Check sheet for the modelled part. Datum: model origin and axes. Units: mm. Face numbers are marked on the shaded views. Round coordinates to 2 decimals unless told otherwise and drop trailing zeros. Order: outer loops, then holes, each group sorted by start corner. A loop starts at its lowest first (then second) coordinate and runs counter-clockwise, first axis right, second up.
from build123d import *

# Parameters (mm, degrees)
SKETCH1_R           = 62.5
SKETCH1_R_2         = 33.5
BOSS_EXTRUDE1_DEPTH = 30
SKETCH2_W           = 16
SKETCH2_H           = 6.75
CUT_EXTRUDE2_DEPTH  = 6
SKETCH3_R           = 51
SKETCH3_R_2         = 45
CUT_EXTRUDE3_DEPTH  = 10.5
SKETCH6_W           = 7.5
SKETCH6_H           = 4.25
CUT_EXTRUDE4_DEPTH  = 8
CUT_EXTRUDE5_START  = -13.375
SKETCH8_R           = 2
CUT_EXTRUDE5_DEPTH  = 60.125
CIRPATTERN1_COUNT   = 6


with BuildPart() as part:
    # Sketch1 → Boss-Extrude1 (new body)
    with BuildSketch(Plane(origin=(0, 0, 0), x_dir=(1, 0, 0), z_dir=(0, 1, 0))):
        Circle(SKETCH1_R)
        Circle(SKETCH1_R_2, mode=Mode.SUBTRACT)
    extrude(amount=BOSS_EXTRUDE1_DEPTH)

    # Sketch2 → Cut-Extrude2 (cut)
    with BuildSketch(Plane(origin=(0, 30, 0), x_dir=(1, 0, 0), z_dir=(0, 1, 0))):
        with Locations((48, 0)):
            Rectangle(SKETCH2_W, SKETCH2_H)
        Polygon((22.922835738, -32.953516151), (17.077164262, -36.328516151), (25.077164262, -50.184922612), (30.922835738, -46.809922612), align=None)
        Polygon((-17.077164262, -36.328516151), (-22.922835738, -32.953516151), (-30.922835738, -46.809922612), (-25.077164262, -50.184922612), align=None)
        with Locations((-48, 0)):
            Rectangle(SKETCH2_W, SKETCH2_H)
        Polygon((-22.922835738, 32.953516151), (-17.077164262, 36.328516151), (-25.077164262, 50.184922612), (-30.922835738, 46.809922612), align=None)
        Polygon((17.077164262, 36.328516151), (22.922835738, 32.953516151), (30.922835738, 46.809922612), (25.077164262, 50.184922612), align=None)
    extrude(amount=-CUT_EXTRUDE2_DEPTH, mode=Mode.SUBTRACT)

    # Sketch3 → Cut-Extrude3 (cut)
    with BuildSketch(Plane(origin=(0, 30, 0), x_dir=(1, 0, 0), z_dir=(0, 1, 0))):
        Circle(SKETCH3_R)
        Circle(SKETCH3_R_2, mode=Mode.SUBTRACT)
    extrude(amount=-CUT_EXTRUDE3_DEPTH, mode=Mode.SUBTRACT)

    # Sketch6 → Cut-Extrude4 (cut)
    with BuildSketch(Plane(origin=(0, 19.5, 0), x_dir=(1, 0, 0), z_dir=(0, 1, 0))):
        with Locations((0, 48)):
            Rectangle(SKETCH6_W, SKETCH6_H)
        Polygon((41.534523365, 28.310095264), (37.853915399, 26.185095264), (41.603915399, 19.689904736), (45.284523365, 21.814904736), align=None)
        Polygon((45.284523365, -21.814904736), (41.603915399, -19.689904736), (37.853915399, -26.185095264), (41.534523365, -28.310095264), align=None)
        with Locations((0, -48)):
            Rectangle(SKETCH6_W, SKETCH6_H)
        Polygon((-41.534523365, -28.310095264), (-37.853915399, -26.185095264), (-41.603915399, -19.689904736), (-45.284523365, -21.814904736), align=None)
        Polygon((-45.284523365, 21.814904736), (-41.603915399, 19.689904736), (-37.853915399, 26.185095264), (-41.534523365, 28.310095264), align=None)
    extrude(amount=-CUT_EXTRUDE4_DEPTH, mode=Mode.SUBTRACT)

    # Sketch8 → Cut-Extrude5 (cut)
    with BuildSketch(Plane.XY.offset(-50.125).offset(CUT_EXTRUDE5_START)):
        with Locations((0, 15.5)):
            Circle(SKETCH8_R)
    cut_extrude5 = extrude(amount=CUT_EXTRUDE5_DEPTH, mode=Mode.SUBTRACT)

    # CirPattern1: Cut-Extrude5 ×6 about axis
    cirpattern1_axis = Axis((0, 19.5, 0), (0, 1, 0))
    for i in range(1, CIRPATTERN1_COUNT):
        add(cut_extrude5.rotate(cirpattern1_axis, i * 360 / CIRPATTERN1_COUNT), mode=Mode.SUBTRACT)


solid = part.part
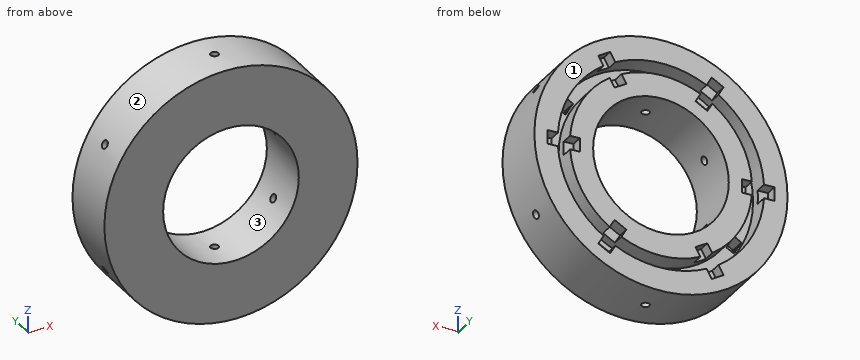
1) Sectioned sample at C-C on y = 8. Record the cut outline in (x, z).
2) Sectioned sample at B-B on x = 11. Record the cut outline in (y, z), and give its area (3 significant figures).
3) Sectioned sample at D-D on y = 15.5. Count the separate pieces of the cut face and the enclosed holes in it, and give its area (3 significant figures).
4) Gauge pin test, flat ends, axial feed: pin 1 (1 mm diameter, centred on x = -35.5, y = 27, fed in from -Z); pin 2 (5 mm diameter, centred on y = 12, z = -25.5, fed in from -X); pin 3 (2.5 mm diameter, centred on x = -25.5, z = -45.5, fed in from +Y). Record the tip position at first contact, or that the pin passes through.
5) Draft check along X on the marked faces 1, 2 and 3. Enter one of: pulls with the +X half, pulls with the -X half, needs draft (parallel to the pull), parting line crosses it, or undercut.
6) Sectioned sample at A-A on z = 0. Record the cut outline in (x, y).
7) Scan lines: line 1 (X direction, y = 22, z = 0); line 2 (Y direction, x = 0, z = -58). Record each from-to range of solid material in increasing order.
Values found:
1. outline: circle Ø125 at (0, 0); hole circle Ø67 at (0, 0)
2. outline: (0, -61.52) - (30, -61.52) - (30, -49.8) - (19.5, -49.8) - (19.5, -43.63) - (30, -43.63) - (30, -31.64) - (0, -31.64) - close; (0, 31.64) - (30, 31.64) - (30, 43.63) - (19.5, 43.63) - (19.5, 49.8) - (30, 49.8) - (30, 61.52) - (0, 61.52) - close
2. area: 1,660 mm2
3. separate pieces: 6
3. enclosed holes: 0
3. area: 7,960 mm2
4. pin 1: stops at z = -51.78
4. pin 2: stops at x = -58.11
4. pin 3: stops at y = 24
5. face 1: needs draft
5. face 2: parting line crosses it
5. face 3: undercut
6. outline: (-62.5, 0) - (-33.5, 0) - (-33.5, 30) - (-40, 30) - (-40, 24) - (-45, 24) - (-45, 19.5) - (-51, 19.5) - (-51, 24) - (-56, 24) - (-56, 30) - (-62.5, 30) - close; (33.5, 0) - (62.5, 0) - (62.5, 30) - (56, 30) - (56, 24) - (51, 24) - (51, 19.5) - (45, 19.5) - (45, 24) - (40, 24) - (40, 30) - (33.5, 30) - close
7. line 1: x = -62.5 to -51, -45 to -33.5, 33.5 to 45, 51 to 62.5
7. line 2: y = 0 to 13.5, 17.5 to 30
